Autodesk Inventor part; units mm, degrees
ref_plane "YZ Plane" through (0, 0, 0) normal (1, 0, 0) x (0, 1, 0)
ref_plane "XZ Plane" through (0, 0, 0) normal (0, 1, 0) x (-1, 0, 0)
ref_plane "XY Plane" through (0, 0, 0) normal (0, 0, 1) x (1, 0, 0)
sketch "スケッチ1" plane through (0, 0, 0) normal (0, 0, 1) x (1, 0, 0)
  line L0 (0, 0) -> (60, 0)
  line L1 (60, 0) -> (60, 60)
  line L2 (60, 60) -> (0, 60)
  line L3 (0, 60) -> (0, 0)
  dimension "d0" = 60
  dimension "d1" = 60
extrude "押し出し1" add sketch "スケッチ1" along normal blind 10
sketch "スケッチ2" plane through (0, 0, 10) normal (0, 0, 1) x (1, 0, 0)
  line L0 (60, 60) -> (0, 60)
  line L1 (60, 0) -> (60, 60)
  line L2 (0, 0) -> (60, 0)
  line L3 (30, 60) -> (30, 0)
  point P0 (35, 55)
  point P1 (55, 35)
  point P2 (55, 25)
  point P3 (35, 5)
  point P4 (25, 55)
  point P5 (5, 35)
  point P6 (5, 25)
  point P7 (25, 5)
  dimension "d4" = 5
  dimension "d5" = 5
  dimension "d6" = 5
  dimension "d7" = 5
  dimension "d8" = 25
  dimension "d9" = 25
  dimension "d10" = 25
  dimension "d11" = 25
hole "穴1" at (35, 55, 10) at (55, 35, 10) at (55, 25, 10) at (35, 5, 10) at (25, 55, 10) at (5, 35, 10) at (5, 25, 10) at (25, 5, 10) direction (0, 0, -1) diameter 3.5 end through all
sketch "スケッチ8" plane through (0, 0, 10) normal (0, 0, 1) x (1, 0, 0)
  line L0 (60, 60) -> (0, 60)
  line L1 (30, 60) -> (30, 0)
  line L2 (0, 0) -> (60, 0)
  line L3 (0, 60) -> (0, 0)
  line L4 (0, 30) -> (60, 30)
  line L5 (60, 0) -> (60, 60)
  point P0 (24, 40)
  point P1 (24, 20)
  point P2 (36, 40)
  point P3 (36, 20)
  dimension "d24" = 12
  dimension "d25" = 20
  dimension "d28" = 20
  dimension "d31" = 12
hole "穴2" at (24, 40, 10) at (24, 20, 10) at (36, 40, 10) at (36, 20, 10) direction (0, 0, -1) diameter 1.567 end through all
properties part number "土台"
Could you check a few things on this model? Use its own coordinates, in mm. Coordinates: 2 decimals unless noted, no trailing zeros. Loops run counter-clockwise (first coordinate to the right, second up) from the corner with the lowest first, then second, coordinate; pieces in that order, holes last. Notation, with made-up numbers: (1, -24) -> (23, -24) arc R20 ccw to (23, 3) -> close; hole circle Ø5 at (9.5, 82). An arc over 180 degrees is marked (long way). Answer in a Markdown table with one row per item.
(1) Imagine slicing it at C-C (x = 5). List the corners of the cut face in (y, z) for me, plus the area to 3 significant figures.
Results found:
| item | result |
|---|---|
| outline | (0, 0) -> (23.25, 0) -> (23.25, 10) -> (0, 10) -> close; (26.75, 0) -> (33.25, 0) -> (33.25, 10) -> (26.75, 10) -> close; (36.75, 0) -> (60, 0) -> (60, 10) -> (36.75, 10) -> close |
| area | 530 mm^2 |
(2) If I drill on probe 1 along Y at (x, z) = (55, 7.75); probe 2 along X at (y, z) = (40, 6), over which ranges is the centre line in solid material (lowest first)?
Results found:
| item | result |
|---|---|
| probe 1 | y = 0 to 23.25, 26.75 to 33.25, 36.75 to 60 |
| probe 2 | x = 0 to 23.22, 24.78 to 35.22, 36.78 to 60 |
(3) Imagine slicing it at D-D (x = 24). List the corners of the cut face in (y, z) for me.
Results found:
| item | result |
|---|---|
| outline | (0, 0) -> (3.56, 0) -> (3.56, 10) -> (0, 10) -> close; (6.44, 0) -> (19.22, 0) -> (19.22, 10) -> (6.44, 10) -> close; (20.78, 0) -> (39.22, 0) -> (39.22, 10) -> (20.78, 10) -> close; (40.78, 0) -> (53.56, 0) -> (53.56, 10) -> (40.78, 10) -> close; (56.44, 0) -> (60, 0) -> (60, 10) -> (56.44, 10) -> close |
(4) Will these pins go through, and if not, where does the flat tip stop? pin 1 Ø2 at (x, y) = (36, 40) entering from +Z; pin 2 Ø1.4 at (x, y) = (36, 20) entering from +Z.
Results found:
| item | result |
|---|---|
| pin 1 | stops at z = 10 |
| pin 2 | passes through |
(5) Imagine slicing it at A-A (y = 35). List the corners of the cut face in (x, z) for me, plus the area to 3 significant figures.
Results found:
| item | result |
|---|---|
| outline | (0, 0) -> (3.25, 0) -> (3.25, 10) -> (0, 10) -> close; (6.75, 0) -> (53.25, 0) -> (53.25, 10) -> (6.75, 10) -> close; (56.75, 0) -> (60, 0) -> (60, 10) -> (56.75, 10) -> close |
| area | 530 mm^2 |
(6) Imagine slicing it at B-B (z = 9.25). Give the number of separate pieces and of enclosed holes in the cut face, plus the area to 3 significant figures.
Results found:
| item | result |
|---|---|
| separate pieces | 1 |
| enclosed holes | 12 |
| area | 3,520 mm^2 |
(7) Thinking about a two-plate mould opening in Y: for faces 1 (the face through (30, 30, 0)), 2 (the face through (6.06, 36.39, 4.93)), 3 (the face through (30, 60, 5)), which applies, released by +Y, released by -Y, zero draft, split by the parting line, or undercut?
Results found:
| item | result |
|---|---|
| face 1 | zero draft |
| face 2 | undercut |
| face 3 | released by +Y |
